Geometry: see drawing. Coordinates: mm, zero at the bounding-box minimum. A direction names the side the tool comes from. Coordinates: 2 decimals unless noted, no trailing zeros. Write each loop counter-clockwise with the first axis right and the second up, starting at its lowest first coordinate (ties: lowest second). Pieces come first, ordered by that corner, then holes. Notation, with made-up numbers: M 39,31.5 L 54,31.5 A11 cw 54,50.5 Z; hole C 40,10.25 d2. An arc over 180 degrees is marked long. Write item = value, one per line. Start each with the question number.
1. Section query D-D (y = 21). Output: boundary loops of the cut face in (x, z) (1 decimal), then the cut area to 3 significant figures.
2. Pin query (flat end, axial travel): pin 1 Ø10 at (y, z) = (31.96, 43.71) entering from +X; pin 2 Ø8 at (x, z) = (57, 2.5) entering from -Y. Return the tip coordinate at first contact, or that it passes through.
3. Line query: line 1 along Z through (x, y) = (17, 13.5); line 2 along X through (y, z) = (17.5, 31) (1 decimal); line 3 along X through (y, z) = (12.5, 81.5) (1 decimal). Output: solid intervals per line, ascending.
4. Section query C-C (y = 43). Output: boundary loops of the cut face in (x, z) (1 decimal).
5. Access query for the marked faces 5 and 6. Directions: +Z, -Z, +X, -X, +Y, -Y. A direction counts if a zero-diameter tool reaches every point of the face in a straight line with its end or side. Return the directions, or none.
6. Pull-direction query (X, two-part tool) for the marked faces 1, 2, 3 and 4; classes: pulls with the +X half, pulls with the -X half, needs draft (parallel to the pull), parting line crosses it, or undercut.
7. Section query A-A (x = 88.5). Output: boundary loops of the cut face in (y, z) (1 decimal), then the cut area to 3 significant figures.
8. Section query B-B (z = 70). Output: boundary loops of the cut face in (x, y) (1 decimal), then the cut area to 3 significant figures.
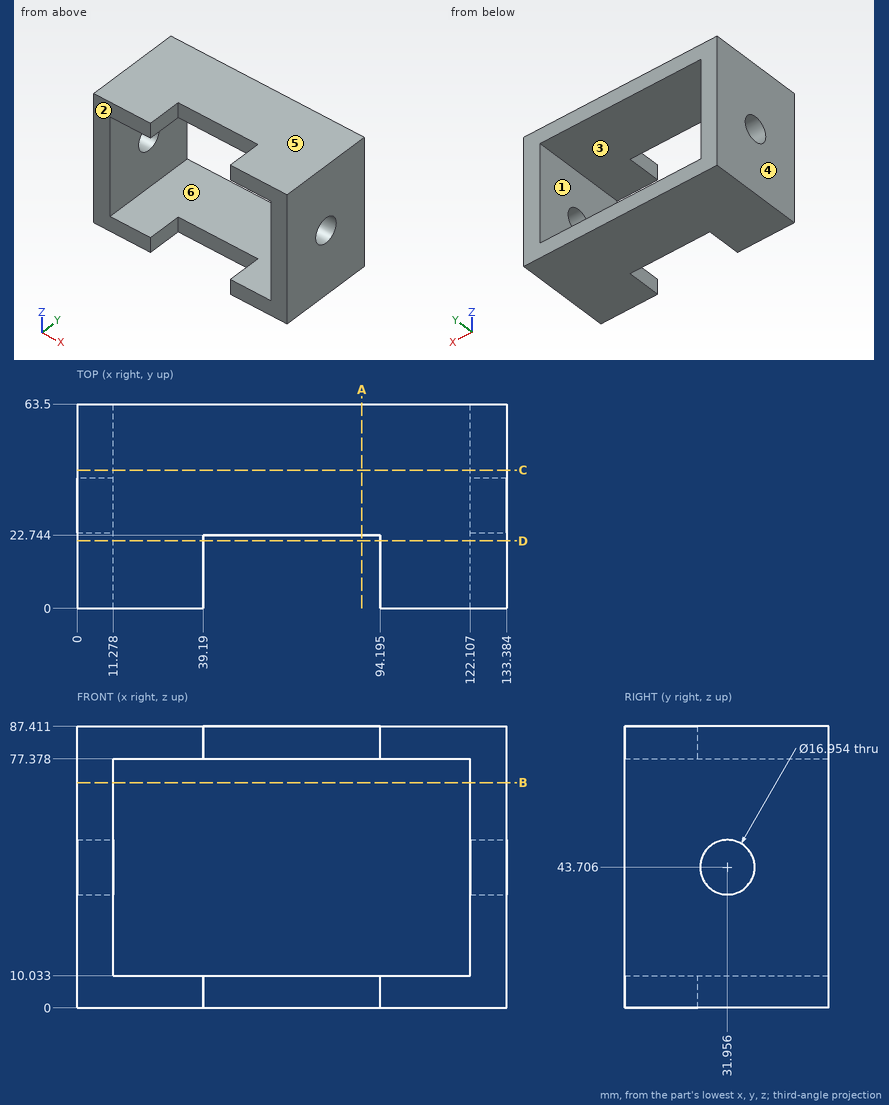
Results are:
q1.outline = M 0,0 L 39.2,0 L 39.2,10 L 11.3,10 L 11.3,77.4 L 39.2,77.4 L 39.2,87.4 L 0,87.4 Z; M 94.2,0 L 133.4,0 L 133.4,87.4 L 94.2,87.4 L 94.2,77.4 L 122.1,77.4 L 122.1,10 L 94.2,10 Z
q1.area = 3,090 mm^2
q2.pin_1 = through
q2.pin_2 = 22.74
q3.line_1 = 0 to 10.03, 77.38 to 87.41
q3.line_2 = 0 to 11.3, 122.1 to 133.4
q3.line_3 = 0 to 39.2, 94.2 to 133.4
q4.outline = M 0,0 L 133.4,0 L 133.4,87.4 L 0,87.4 Z; hole M 11.3,10 L 122.1,10 L 122.1,77.4 L 11.3,77.4 Z
q5.face_5 = +Z, +X, -X, +Y, -Y
q5.face_6 = +Y, -Y
q6.face_1 = undercut
q6.face_2 = needs draft
q6.face_3 = undercut
q6.face_4 = pulls with the -X half
q7.outline = M 22.7,0 L 63.5,0 L 63.5,10 L 22.7,10 Z; M 22.7,77.4 L 63.5,77.4 L 63.5,87.4 L 22.7,87.4 Z
q7.area = 818 mm^2
q8.outline = M 0,0 L 11.3,0 L 11.3,63.5 L 0,63.5 Z; M 122.1,0 L 133.4,0 L 133.4,63.5 L 122.1,63.5 Z
q8.area = 1,430 mm^2
